from build123d import *

# Parameters (mm, degrees)
F0_R     = 15
F0_R_2   = 8
F0_R_3   = 1.5
F1_DEPTH = 40
F2_DEPTH = 16
F3_SIZE2 = 35
F3_SIZE  = 15


with BuildPart() as f1:
    # F0 (on Top) → F1 (new body)
    with BuildSketch(Plane.XY):
        Circle(F0_R)
        Circle(F0_R_2, mode=Mode.SUBTRACT)
        Circle(F0_R_2)
        Circle(F0_R_3, mode=Mode.SUBTRACT)
        Circle(F0_R_3)
    extrude(amount=F1_DEPTH)

    # F0 (on Top) → F2 (cut)
    with BuildSketch(Plane.XY):
        Circle(F0_R_2)
        Circle(F0_R_3, mode=Mode.SUBTRACT)
        Circle(F0_R_3)
    extrude(amount=F2_DEPTH, mode=Mode.SUBTRACT)

    # F3
    f3_edges = [f1.edges().sort_by_distance(p)[0] for p in [
        (-15, 0, 40),
    ]]
    f3_side = f1.faces().sort_by_distance((0, 0, 40))[0]
    chamfer(f3_edges, length=F3_SIZE, length2=F3_SIZE2, reference=f3_side)


solid = f1.part
Source: CAD feature listing. Evaluate the final solid. Frame: model axes, mm. A direction names the side the tool comes from. Give positions to 0.01 mm unless a question says otherwise; leave off trailing zeros. Loops run counter-clockwise (first coordinate to the right, second up) from the corner with the lowest first, then second, coordinate; pieces in that order, holes last. Notation, with made-up numbers: (16, -6.5) -> (38, -6.5) arc R24 cw to (38, 29.5) -> close; hole circle Ø3 at (79, 24.5). An arc over 180 degrees is marked (long way). Use a Markdown table: item, result. Add a question column.
1) Section query A-A, the plane z = 29.5. Return the cut outline in (x, y), then the cut area to 3 significant figures.
2) Reachability of faces 1 (the face through (-1.73, -7.81, 7.89)), 2 (the face through (-1.29, -5.8, 26.14)) from +Z, -Z, +X, -X, +Y, -Y: full face, straight path, thin tool, end or side. Return the list, or none.
3) Section query C-C, the plane z = 9. Return the cut outline in (x, y).
4) Section query B-B, the plane z = 3.5. Return the cut outline in (x, y).
5) Section query D-D, the plane z = 34. Return the cut outline in (x, y).
6) First-contact query: pin 1 (8 mm diameter, centred on x = -10, z = 12, fed in from -Y); pin 2 (3 mm diameter, centred on y = -5.5, z = 23, fed in from +X); pin 3 (1.5 mm diameter, centred on y = 6, z = 25, fed in from -X). Flat tips, straight axial feed; report the tip coordinate or a pass-through.
7) Line query: line 1 along Y through (x, z) = (0, 4.25); line 2 along Y through (x, z) = (0, 8); line 3 along Z through (x, y) = (-5, 3). Output: solid intervals per line, ascending. Write a range as [from, to].
8) Pull-direction query (X, two-part tool) for faces 3 (the face through (6, -6, 0)), 4 (the face through (-14.985, 0.66, 2.465)), 5 (the face through (0, 0, 16)); classes: +X half, -X half, draft (parallel to the pull), parting line (faces both ways), or undercut.
Numbers:
| question | item | result |
|---|---|---|
| 1 | outline | circle Ø9 at (0, 0) |
| 1 | area | 63.6 mm2 |
| 2 | face 1 | -Z |
| 2 | face 2 | +Z |
| 3 | outline | circle Ø26.57 at (0, 0); hole circle Ø16 at (0, 0) |
| 4 | outline | circle Ø30 at (0, 0); hole circle Ø16 at (0, 0) |
| 5 | outline | circle Ø5.14 at (0, 0) |
| 6 | pin 1 | stops at y = -11.12 |
| 6 | pin 2 | stops at x = 6.35 |
| 6 | pin 3 | stops at x = -3.85 |
| 7 | line 1 | y = [-15, -8], [8, 15] |
| 7 | line 2 | y = [-13.71, -8], [8, 13.71] |
| 7 | line 3 | z = [16, 26.39] |
| 8 | face 3 | draft |
| 8 | face 4 | parting line |
| 8 | face 5 | undercut |
